Design review of the part built by this model. Coordinates are the model's own, in mm. A direction names the side the tool comes from. Coordinates: 2 decimals unless noted, no trailing zeros. Loops run counter-clockwise (first coordinate to the right, second up) from the corner with the lowest first, then second, coordinate; pieces in that order, holes last. Notation, with made-up numbers: (29.5, 12.5) -> (38.5, 12.5) arc R6 cw to (38.5, 23.5) -> close; hole circle Ø5 at (30.5, -18). An arc over 180 degrees is marked (long way). Use CSV: the item, a comma, the result in double quotes.
```python
from build123d import *

# Parameters (mm, degrees)
SKETCH1_R           = 4
BOSS_EXTRUDE1_DEPTH = 8
SKETCH2_W           = 30
SKETCH2_H           = 10
BOSS_EXTRUDE2_DEPTH = 100
FILLET1_R           = 10
SKETCH5_W           = 45
SKETCH5_H           = 25
SKETCH5_R           = 4
BOSS_EXTRUDE4_DEPTH = 10


with BuildPart() as part:
    # Sketch1 → Boss-Extrude1 (new body)
    with BuildSketch(Plane.XY):
        with BuildLine():
            Line((15, 30), (15, -30))
            ThreePointArc((15, -30), (0, -45), (-15, -30))
            Line((-15, -30), (-15, 30))
            ThreePointArc((-15, 30), (0, 45), (15, 30))
        make_face()
        with Locations((0, 30)):
            Circle(SKETCH1_R, mode=Mode.SUBTRACT)
        with Locations((0, -30)):
            Circle(SKETCH1_R, mode=Mode.SUBTRACT)
    extrude(amount=BOSS_EXTRUDE1_DEPTH)

    # Sketch2 → Boss-Extrude2 (add)
    with BuildSketch(Plane.XY):
        Rectangle(SKETCH2_W, SKETCH2_H)
    extrude(amount=BOSS_EXTRUDE2_DEPTH)

    # Fillet1
    fillet1_edges = [part.edges().sort_by_distance(p)[0] for p in [
        (0, 5, 8),
        (0, -5, 8),
    ]]
    fillet(fillet1_edges, radius=FILLET1_R)

    # Sketch5 → Boss-Extrude4 (add)
    with BuildSketch(Plane(origin=(0, 5, 0), x_dir=(1, 0, 0), z_dir=(0, 1, 0))):
        with Locations((7.5, -112.5)):
            Rectangle(SKETCH5_W, SKETCH5_H)
        with Locations((20, -112.5)):
            Circle(SKETCH5_R, mode=Mode.SUBTRACT)
    extrude(amount=-BOSS_EXTRUDE4_DEPTH)


solid = part.part
```
Item 1: Clearance check with flat-ended pins moving along their axes: pin 1 (10 mm diameter, centred on x = 4.5, z = 38, fed in from +Y); pin 2 (15 mm diameter, centred on x = -4, y = -25, fed in from +Z); pin 3 (3 mm diameter, centred on x = 26, y = -0.5, fed in from -Z). State where each tip first meets the part, or that it passes through.
Checked values:
pin 1,"y = 5"
pin 2,"z = 8"
pin 3,"z = 100"
Item 2: Add section B-B (y = -3). Give the boundary of the cut face in (x, z), then the cut area to 3 significant figures.
Checked values:
outline,"(-15, 0) -> (15, 0) -> (15, 100) -> (30, 100) -> (30, 125) -> (-15, 125) -> close; hole circle Ø8 at (20, 112.5)"
area,"4,070 mm^2"
Item 3: Add section A-A (x = 0). Give the boundary of the cut face in (y, z), then the cut area to 3 significant figures.
Checked values:
outline,"(-45, 0) -> (-34, 0) -> (-34, 8) -> (-45, 8) -> close; (-26, 0) -> (26, 0) -> (26, 8) -> (15, 8) arc R10 cw to (5, 18) -> (5, 125) -> (-5, 125) -> (-5, 18) arc R10 cw to (-15, 8) -> (-26, 8) -> close; (34, 0) -> (45, 0) -> (45, 8) -> (34, 8) -> close"
area,"1,800 mm^2"
Item 4: Add section C-C (z = 112.5). Give the boundary of the cut face in (x, y), then the cut area to 3 significant figures.
Checked values:
outline,"(-15, -5) -> (16, -5) -> (16, 5) -> (-15, 5) -> close; (24, -5) -> (30, -5) -> (30, 5) -> (24, 5) -> close"
area,"370 mm^2"
Item 5: Draft analysis for pull direction Z (two halves, no side actions). For faces 4 (the face through (22, 0, 100)), 5 (the face through (2, 5, 71)), 6 (the face through (19.479, 0.07, 108.534)), state which applies: pulls with the +Z half, pulls with the -Z half, needs draft (parallel to the pull), parting line crosses it, or undercut.
Checked values:
face 4,"pulls with the -Z half"
face 5,"needs draft"
face 6,"undercut"
Item 6: Machinability: for faces 1 (the face through (-3, 27, 8)), 2 (the face through (2, -5, 71)), 3 (the face through (15, 0, 39)), which of the approach directions +Z, -Z, +X, -X, +Y, -Y give a long, thin tool a straight path to every point of the face, cutting with its end or side? Answer none if there is none.
Checked values:
face 1,"+Z, +X, -X, +Y"
face 2,"+Z, +X, -X, -Y"
face 3,"-Z, +X, +Y, -Y"
Item 7: To check wall thickness, follow line 1 along Y through (x, z) = (0, 4.75); line 2 along X through (y, z) = (1.25, 112.5); line 3 along Z through (x, y) = (20, -2). State the ranges of each line that lie inside material, in increasing order.
Checked values:
line 1,"-45 to -34, -26 to 26, 34 to 45"
line 2,"-15 to 16, 24 to 30"
line 3,"100 to 108.5, 116.5 to 125"
Item 8: Add section D-D (x = 20). Give the boundary of the cut face in (y, z), then the cut area to 3 significant figures.
Checked values:
outline,"(-5, 100) -> (5, 100) -> (5, 108.5) -> (-5, 108.5) -> close; (-5, 116.5) -> (5, 116.5) -> (5, 125) -> (-5, 125) -> close"
area,"170 mm^2"
